Autodesk Inventor part; units mm, degrees
ref_plane "YZ Plane" through (0, 0, 0) normal (1, 0, 0) x (0, 1, 0)
ref_plane "XZ Plane" through (0, 0, 0) normal (0, 1, 0) x (-1, 0, 0)
ref_plane "XY Plane" through (0, 0, 0) normal (0, 0, 1) x (1, 0, 0)
sketch "スケッチ2" plane through (0, 0, 0) normal (0, 0, 1) x (1, 0, 0)
  circle A0 centre (0, 0) radius 10.1 construction
  circle A1 centre (25.3202, -9.9362) radius 17.1 construction
  circle A2 centre (110.4743, -16.4118) radius 28.1 construction
  circle A3 centre (62.4131, -12.7569) radius 20.1 construction
  circle A4 centre (-21.6908, -16.4118) radius 17.1 construction
  circle A5 centre (-105.5257, -16.4118) radius 28.1 construction
  line L0 (-170.915, -81.4118) -> (490.0044, -81.4118)
  line L1 (-105.5257, -16.4118) -> (-21.6908, -16.4118) construction
  line L2 (110.4743, -16.4118) -> (25.3202, -9.9362) construction
  line L3 (110.4743, -16.4118) -> (104.1501, -0.632)
  line L4 (104.1501, -0.632) -> (95.5937, 20.7173) construction
  line L5 (95.5937, 20.7173) -> (70.4743, -10.4118) construction
  line L6 (70.4743, -10.4118) -> (110.4743, -16.4118) construction
  line L7 (-137.6819, 53.5882) -> (165.8186, 53.5882)
  line L8 (25.3202, -9.9362) -> (108.6869, 8.5882) construction
  line L9 (25.3202, -9.9362) -> (102.5386, -46.4118) construction
  line L10 (25.3202, -9.9362) -> (5.9362, 53.5882) construction
  line L11 (5.9362, 53.5882) -> (127.6431, 30.2622)
  line L12 (127.6431, 30.2622) -> (110.4743, -16.4118) construction
  line L13 (102.5386, -46.4118) -> (118.0681, 0.8329) construction
  line L14 (118.0681, 0.8329) -> (5.9362, 53.5882) construction
  line L15 (108.6869, 8.5882) -> (129.8583, 53.5882) construction
  line L16 (129.8583, 53.5882) -> (5.9362, 53.5882) construction
  line L17 (119.2726, 31.0882) -> (366.4441, 68.5882) construction
  line L18 (119.0587, 6.9252) -> (362.0213, 65.8249) construction
  line L19 (110.3034, -22.7894) -> (351.0624, 44.5537) construction
  line L20 (127.6431, 30.2622) -> (4.1927, 19.4617) construction
  circle A6 centre (80.4743, 23.124) radius 3 construction
  circle A7 centre (80.4743, 23.124) radius 1.5
  arc A8 (79.801, 27.5733) -> (76.162, 24.4099) centre (80.4743, 23.124) ccw
  circle A9 centre (70.4743, -10.4118) radius 1.5
  arc A10 (66.162, -9.1259) -> (69.4242, -14.7876) centre (70.4743, -10.4118) ccw
  circle A11 centre (150.4743, 0.5882) radius 1.5
  arc A12 (152.5623, -3.3981) -> (154.0408, 3.3323) centre (150.4743, 0.5882) ccw
  circle A13 centre (127.6431, 30.2622) radius 1.5
  arc A14 (131.2816, 32.9102) -> (126.9698, 34.7115) centre (127.6431, 30.2622) ccw
  circle A15 centre (110.4743, -16.4118) radius 5
  arc A16 (108.6075, -24.1909) -> (114.1862, -23.4986) centre (110.4743, -16.4118) ccw
  line L21 (76.162, 24.4099) -> (66.162, -9.1259)
  line L22 (69.4242, -14.7876) -> (108.6075, -24.1909)
  line L23 (114.1862, -23.4986) -> (152.5623, -3.3981)
  line L24 (154.0408, 3.3323) -> (131.2097, 33.0062)
  line L25 (126.9698, 34.7115) -> (79.801, 27.5733)
  circle A17 centre (-145.5257, 0.5882) radius 1.5
  arc A18 (-149.0922, 3.3323) -> (-147.6136, -3.3981) centre (-145.5257, 0.5882) ccw
  circle A19 centre (-105.5257, -16.4118) radius 5
  arc A20 (-109.2375, -23.4986) -> (-103.6588, -24.1909) centre (-105.5257, -16.4118) ccw
  circle A21 centre (-65.5257, -10.4118) radius 1.5
  arc A22 (-64.4756, -14.7876) -> (-61.2133, -9.1259) centre (-65.5257, -10.4118) ccw
  circle A23 centre (0, 0) radius 20.05 construction
  circle A24 centre (110.4743, -16.4118) radius 30.1 construction
  circle A25 centre (62.4131, -12.7569) radius 22.1 construction
  circle A26 centre (25.3202, -9.9362) radius 19.1 construction
  circle A27 centre (0, 0) radius 12.1 construction
  circle A28 centre (-21.6908, -16.4118) radius 19.1 construction
  circle A29 centre (-105.5257, -16.4118) radius 30.1 construction
  circle A30 centre (0, 0) radius 20.55 construction
  circle A31 centre (95.5937, 20.7173) radius 4.025 construction
  circle A32 centre (95.5937, 20.7173) radius 6.025 construction
  circle A33 centre (-75.5257, 23.124) radius 1.5
  arc A34 (-71.2133, 24.4099) -> (-74.8523, 27.5733) centre (-75.5257, 23.124) ccw
  circle A35 centre (-122.6945, 30.2622) radius 1.5
  arc A36 (-122.0212, 34.7115) -> (-126.261, 33.0062) centre (-122.6945, 30.2622) ccw
  line L26 (-126.261, 33.0062) -> (-149.0922, 3.3323)
  line L27 (-147.6136, -3.3981) -> (-109.2375, -23.4986)
  line L28 (-103.6588, -24.1909) -> (-64.4756, -14.7876)
  line L29 (-61.2133, -9.1259) -> (-71.2133, 24.4099)
  line L30 (-74.8523, 27.5733) -> (-122.0212, 34.7115)
  circle A37 centre (14, -17.4118) radius 2.2921 construction
  circle A38 centre (-14, -17.4118) radius 2.2921 construction
  circle A39 centre (-14, -17.4118) radius 14 construction
  circle A40 centre (14, -17.4118) radius 14 construction
  line L31 (-170.6512, -31.4118) -> (202.8656, -31.4118)
  line L32 (5.9362, 53.5882) -> (-38.6574, 35.6253) construction
  line L33 (5.9362, 53.5882) -> (-26.7676, 18.3503) construction
  circle A41 centre (5.9362, 53.5882) radius 1.5
  arc A42 (9.9603, 55.6024) -> (4.2549, 57.7623) centre (5.9362, 53.5882) ccw
  line L34 (-21.6908, -16.4118) -> (-99.9742, 13.5882) construction
  line L35 (-21.6908, -16.4118) -> (-101.7113, -41.4118) construction
  line L36 (9.9603, 55.6024) -> (33.1621, 9.2488)
  circle A43 centre (-47.0055, 32.2626) radius 1.5
  arc A44 (-48.6869, 36.4367) -> (-50.4404, 29.3554) centre (-47.0055, 32.2626) ccw
  line L37 (4.2549, 57.7623) -> (-48.6869, 36.4367)
  line L38 (-50.4404, 29.3554) -> (-38.6655, 15.4431)
  circle A45 centre (29.1381, 7.2346) radius 3 construction
  circle A46 centre (-84.8661, 5.2713) radius 4.5 construction
  circle A47 centre (-132.0174, -1.9813) radius 4.5 construction
  line L39 (-132.7015, 2.4664) -> (-85.5502, 9.719) construction
  arc A48 (28.3723, 2.8003) -> (33.1621, 9.2488) centre (29.1381, 7.2346) ccw
  arc A49 (-38.6655, 15.4431) -> (-35.9964, 13.9159) centre (-35.2306, 18.3503) ccw
  line L40 (-35.9964, 13.9159) -> (28.3723, 2.8003)
  circle A50 centre (-38.6574, 35.6253) radius 3 construction
  circle A51 centre (25.3202, -9.9362) radius 4.025 construction
  circle A52 centre (-21.6908, -16.4118) radius 4.025 construction
  circle A53 centre (-35.2306, 18.3503) radius 1.5
  circle A54 centre (29.1381, 7.2346) radius 1.5
  circle A55 centre (-57.813, 39.7705) radius 4.5 construction
  circle A56 centre (-99.304, 63.3152) radius 4.5 construction
  line L41 (5.9362, 53.5882) -> (-32.8159, 25.1361) construction
  circle A57 centre (-58.0056, -24.4791) radius 20.1 construction
  circle A58 centre (-58.0056, -24.4791) radius 22.1 construction
  line L42 (-53.3261, 39.4281) -> (-56.2797, 0.7243) construction
  circle A59 centre (-38.6574, 35.6253) radius 4.5
  dimension "d207" = 9
  dimension "d208" = 9
  dimension "d223" = 9
  dimension "d119" = 20.2
  dimension "d120" = 34.2
  dimension "d121" = 56.2
  dimension "d122" = 40.2
  dimension "d123" = 216
  dimension "d124" = 65
  dimension "d125" = 65
  dimension "d126" = 34.2
  dimension "d127" = 56.2
  dimension "d128" = 17
  dimension "d129" = 23
  dimension "d130" = 40
  dimension "d131" = 40
  dimension "d132" = 6
  dimension "d133" = 135
  dimension "d134" = 25
  dimension "d135" = 30
  dimension "d136" = 5
  dimension "d137" = 2
  dimension "d138" = 250
  dimension "d139" = 150
  dimension "d140" = 250
  dimension "d141" = 250
  dimension "d142" = 123.823
  dimension "d143" = 123.823
  dimension "d144" = 123.823
  dimension "d145" = 6
  dimension "d146" = 3
  dimension "d147" = 9
  dimension "d148" = 3
  dimension "d149" = 9
  dimension "d150" = 3
  dimension "d151" = 9
  dimension "d152" = 40
  dimension "d153" = 17
  dimension "d154" = 3
  dimension "d155" = 9
  dimension "d156" = 10
  dimension "d157" = 3
  dimension "d158" = 3
  dimension "d159" = 9
  dimension "d160" = 40
  dimension "d161" = 17
  dimension "d162" = 10
  dimension "d163" = 3
  dimension "d164" = 3
  dimension "d165" = 9
  dimension "d166" = 40
  dimension "d167" = 6
  dimension "d168" = 40.1
  dimension "d169" = 2
  dimension "d170" = 2
  dimension "d171" = 2
  dimension "d172" = 2
  dimension "d173" = 2
  dimension "d174" = 2
  dimension "d175" = 0.5
  dimension "d176" = 8.05
  dimension "d177" = 2
  dimension "d178" = 3
  dimension "d179" = 9
  dimension "d180" = 3
  dimension "d181" = 9
  dimension "d182" = 46.674
extrude "押し出し2" add sketch "スケッチ2" along normal blind 3 contours A41 L7 L37 A42 L36 | L7 L36 L11 A41 | A59 | A41 L11 L36 A48 L40 A49 L38 A44 L37 L7
equation "\"d126\" = d120"
equation "\"d127\" = d121"
equation "\"d143\" = d142"
equation "\"d144\" = d142"
properties part number "中間外フレーム" material "ポリカーボネート、クリア"
Input: part model. Units: mm. Frame: model coordinates. Coordinates: 2 decimals unless noted, no trailing zeros. Order: outer loops, then holes, each group sorted by start corner. A loop starts at its lowest first (then second) coordinate and runs counter-clockwise, first axis right, second up. Notation, with made-up numbers: (39.5, -12.5) - (81.5, -12.5) arc R16 cw to (81.5, -0.5) - close; hole circle Ø9 at (83, 48.5). An arc over 180 degrees is marked (long way). Put each result on its own line as item: value.
1. Cut plane C-C on y = 21. Return the cut outline in (x, z).
Report:
outline: (-43.37, 0) - (27.28, 0) - (27.28, 3) - (-43.37, 3) - close
2. Contact query for flat-ended pins moving along their axis: pin 1 Ø1.8 at (x, y) = (-35.23, 18.35) entering from -Z; pin 2 Ø1 at (x, z) = (17.5, 2.5) entering from +Y. Output: stop coordinate, or through.
Report:
pin 1: passes through
pin 2: stops at y = 41.54
3. Cut plane A-A on z = 1.1. Return the cut outline in (x, y), then the cut area to 3 significant figures.
Report:
outline: (-50.44, 29.36) - (-38.67, 15.44) arc R4.5 ccw to (-36, 13.92) - (28.37, 2.8) arc R4.5 ccw to (33.16, 9.25) - (9.96, 55.6) arc R4.5 ccw to (4.25, 57.76) - (-48.69, 36.44) arc R4.5 ccw to start; hole circle Ø3 at (-47.01, 32.26); hole circle Ø3 at (-35.23, 18.35); hole circle Ø3 at (5.94, 53.59); hole circle Ø3 at (29.14, 7.23)
area: 2,760 mm2
4. Draft query along Y for faces 1 (the face through (-21.845, 47.249, 1.479)), 2 (the face through (-10, 31, 3)), 3 (the face through (-33.845, 18.925, 1.479)). Return one class per face: pulls with the +Y half, pulls with the -Y half, needs draft (parallel to the pull), parting line crosses it, or undercut.
Report:
face 1: pulls with the +Y half
face 2: needs draft
face 3: undercut
5. Line query: line 1 along X through (y, z) = (17, 1.05); line 2 along Y through (x, z) = (5.5, 2.05); line 3 along Y through (x, z) = (6, 0.8). Output: solid intervals per line, ascending.
Report:
line 1: x = -39.98 to -35.88, -34.58 to 29.28
line 2: y = 6.75 to 52.15, 55.02 to 58.07
line 3: y = 6.66 to 52.09, 55.09 to 58.09
6. Cut plane B-B on x = -17. Return the cut outline in (y, z).
Report:
outline: (10.64, 0) - (49.2, 0) - (49.2, 3) - (10.64, 3) - close
